Here's how the part is built. I have some questions about the finished solid (model axes, mm). Coordinates: 2 decimals unless noted, no trailing zeros. Loops run counter-clockwise (first coordinate to the right, second up) from the corner with the lowest first, then second, coordinate; pieces in that order, holes last. Notation, with made-up numbers: M 32,56 L 58,56 A21 cw 58,76 Z; hole C -28.5,2.5 d7. An arc over 180 degrees is marked long. Use one line per item in the form item = value. Start each with the question number.
(1) Imagine slicing it at C-C, the plane y = 1.45. Please give me the cut outline in (x, z), and give its area (3 significant figures).
(2) Will these pins go through, and if not, where does the flat tip stop? P1, Ø1.5, axis at x = 80, y = 1.5, coming from the +Z side; P2, Ø4, axis at x = 2.75, z = 84.75, coming from the +Y side; P3, Ø1.5, axis at y = 2, z = 51.5, coming from the +X side; P4, Ø1.5, axis at y = 2, z = 49, coming from the -X side.
(3) Please list where these lines run through material, in increasing order: L1, parallel to Z at x = 135.75, y = 1.45; L2, parallel to X at y = 1.55, z = 84.75; L3, parallel to Z at x = 26.15, y = 0.95.
(4) Imagine slicing it at B-B, the plane x = 26.15. Please give me the cut outline in (y, z).
(5) Imagine slicing it at A-A, the plane z = 2.75. Please give me the cut outline in (x, y).
(6) Imagine slicing it at D-D, the plane z = 47.5. Please give me the cut outline in (x, y), and give its area (3 significant figures).
```python
from build123d import *

# Parameters (mm, degrees)
SKETCH1_W           = 138.5
SKETCH1_H           = 87.5
BOSS_EXTRUDE1_DEPTH = 3
SKETCH2_R           = 1.75
CUT_EXTRUDE1_DEPTH  = 4
SKETCH3_W           = 9.5
SKETCH3_H           = 3.25
SKETCH3_W_2         = 3.25
SKETCH3_H_2         = 9.5
BOSS_EXTRUDE2_DEPTH = 3
SKETCH4_R           = 3.75
CUT_EXTRUDE2_DEPTH  = 4


with BuildPart() as part:
    # Sketch1 → Boss-Extrude1 (new body)
    with BuildSketch(Plane(origin=(0, 0, 0), x_dir=(1, 0, 0), z_dir=(0, 1, 0))):
        with Locations((69.25, -43.75)):
            Rectangle(SKETCH1_W, SKETCH1_H)
    extrude(amount=BOSS_EXTRUDE1_DEPTH)

    # Sketch2 → Cut-Extrude1 (cut, through all)
    with BuildSketch(Plane.XZ):
        with Locations((2.75, 84.75)):
            Circle(SKETCH2_R)
        with Locations((135.75, 84.75)):
            Circle(SKETCH2_R)
        with Locations((135.75, 2.75)):
            Circle(SKETCH2_R)
        with Locations((2.75, 2.75)):
            Circle(SKETCH2_R)
    extrude(amount=-CUT_EXTRUDE1_DEPTH, mode=Mode.SUBTRACT)

    # Sketch3 → Boss-Extrude2 (add, through all)
    with BuildSketch(Plane.XZ):
        Polygon((0, 90.75), (-3.25, 90.75), (-3.25, 78), (0, 78), (0, 87.5), align=None)
        with Locations((4.75, 89.125)):
            Rectangle(SKETCH3_W, SKETCH3_H)
        with Locations((-1.625, 4.75)):
            Rectangle(SKETCH3_W_2, SKETCH3_H_2)
        Polygon((9.5, 0), (0, 0), (-3.25, 0), (-3.25, -3.25), (9.5, -3.25), align=None)
        Polygon((138.5, 0), (129, 0), (129, -3.25), (141.75, -3.25), (141.75, 0), align=None)
        with Locations((140.125, 4.75)):
            Rectangle(SKETCH3_W_2, SKETCH3_H_2)
        with Locations((133.75, 89.125)):
            Rectangle(SKETCH3_W, SKETCH3_H)
        Polygon((138.5, 90.75), (138.5, 87.5), (138.5, 78), (141.75, 78), (141.75, 90.75), align=None)
    extrude(amount=-BOSS_EXTRUDE2_DEPTH)

    # Sketch4 → Cut-Extrude2 (cut, through all)
    with BuildSketch(Plane.XZ):
        with Locations((26.15, 47.5)):
            Circle(SKETCH4_R)
        with Locations((26.15, 27.75)):
            Circle(SKETCH4_R)
    extrude(amount=-CUT_EXTRUDE2_DEPTH, mode=Mode.SUBTRACT)


solid = part.part
```
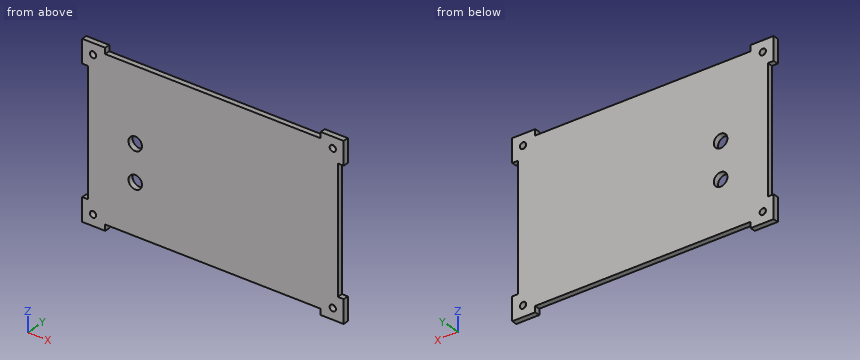
Answer:
q1.outline = M -3.25,-3.25 L 9.5,-3.25 L 9.5,0 L 129,0 L 129,-3.25 L 141.75,-3.25 L 141.75,9.5 L 138.5,9.5 L 138.5,78 L 141.75,78 L 141.75,90.75 L 129,90.75 L 129,87.5 L 9.5,87.5 L 9.5,90.75 L -3.25,90.75 L -3.25,78 L 0,78 L 0,9.5 L -3.25,9.5 Z; hole C 2.75,2.75 d3.5; hole C 2.75,84.75 d3.5; hole C 26.15,27.75 d7.5; hole C 26.15,47.5 d7.5; hole C 135.75,2.75 d3.5; hole C 135.75,84.75 d3.5
q1.area = 12,300 mm²
q2.P1 = 87.5
q2.P2 = 3
q2.P3 = 138.5
q2.P4 = 0
q3.L1 = -3.25 to 1, 4.5 to 83, 86.5 to 90.75
q3.L2 = -3.25 to 1, 4.5 to 134, 137.5 to 141.75
q3.L3 = 0 to 24, 31.5 to 43.75, 51.25 to 87.5
q4.outline = M 0,0 L 3,0 L 3,24 L 0,24 Z; M 0,31.5 L 3,31.5 L 3,43.75 L 0,43.75 Z; M 0,51.25 L 3,51.25 L 3,87.5 L 0,87.5 Z
q5.outline = M -3.25,0 L 1,0 L 1,3 L -3.25,3 Z; M 4.5,0 L 134,0 L 134,3 L 4.5,3 Z; M 137.5,0 L 141.75,0 L 141.75,3 L 137.5,3 Z
q6.outline = M 0,0 L 22.4,0 L 22.4,3 L 0,3 Z; M 29.9,0 L 138.5,0 L 138.5,3 L 29.9,3 Z
q6.area = 393 mm²
